from build123d import *

# Parameters (mm, degrees)
SKETCH1_W           = 54.7
SKETCH1_H           = 54.7
BOSS_EXTRUDE1_DEPTH = 6.35
SKETCH2_W           = 6.35
SKETCH2_H           = 13.5
SKETCH2_H_2         = 6.35
SKETCH2_W_2         = 13.5
CUT_EXTRUDE1_DEPTH  = 40.196524081


with BuildPart() as part:
    # Sketch1 → Boss-Extrude1 (new body)
    with BuildSketch(Plane.XY):
        Rectangle(SKETCH1_W, SKETCH1_H)
    extrude(amount=BOSS_EXTRUDE1_DEPTH)

    # Sketch2 → Cut-Extrude1 (cut, through all)
    with BuildSketch(Plane.XY.offset(6.35)):
        with Locations((-24.175, 14.25)):
            Rectangle(SKETCH2_W, SKETCH2_H)
        with Locations((-24.175, 24.175)):
            Rectangle(SKETCH2_W, SKETCH2_H_2)
        with Locations((-14.25, 24.175)):
            Rectangle(SKETCH2_W_2, SKETCH2_H_2)
        with Locations((14.25, 24.175)):
            Rectangle(SKETCH2_W_2, SKETCH2_H_2)
        with Locations((24.175, 24.175)):
            Rectangle(SKETCH2_W, SKETCH2_H_2)
        with Locations((24.175, 14.25)):
            Rectangle(SKETCH2_W, SKETCH2_H)
        with Locations((24.175, -14.25)):
            Rectangle(SKETCH2_W, SKETCH2_H)
        with Locations((24.175, -24.175)):
            Rectangle(SKETCH2_W, SKETCH2_H_2)
        with Locations((14.25, -24.175)):
            Rectangle(SKETCH2_W_2, SKETCH2_H_2)
        with Locations((-14.25, -24.175)):
            Rectangle(SKETCH2_W_2, SKETCH2_H_2)
        with Locations((-24.175, -24.175)):
            Rectangle(SKETCH2_W, SKETCH2_H_2)
        with Locations((-24.175, -14.25)):
            Rectangle(SKETCH2_W, SKETCH2_H)
    extrude(amount=-CUT_EXTRUDE1_DEPTH, mode=Mode.SUBTRACT)


solid = part.part
Here's how the part is built. I have some questions about the finished solid (model axes, mm). A direction names the side the tool comes from. Give positions to 0.01 mm unless a question says otherwise; leave off trailing zeros. Loops run counter-clockwise (first coordinate to the right, second up) from the corner with the lowest first, then second, coordinate; pieces in that order, holes last. Notation, with made-up numbers: (-21.75, -7) -> (2.25, -7) arc R22 cw to (2.25, 19) -> close; hole circle Ø3 at (55.25, 43.25). An arc over 180 degrees is marked (long way). Answer as a JSON object with one key per item and string values. Group by question number.
Item 1: I need wall thicknesses on L1, parallel to X at y = -11.5, z = 2; L2, parallel to X at y = 22, z = 4.5. Which ranges of each line are inside material? Lowest first, please.
Item 2: Imagine slicing it at B-B on y = 17. Write out the boundary of the cut face in (x, z).
Item 3: On a 3-axis mill with a long thin cutter (end or side, diameter ignored), from which of +Z, -Z, +X, -X, +Y, -Y can I reach the whole of each face in a straight line? I mean faces 1 (the flat face through (14, -21, 3)), 2 (the flat face through (-24, 7.5, 3)), 3 (the flat face through (-14, -21, 3)), 4 (the flat face through (24, 7.5, 3)), 5 (the flat face through (27.35, 0, 3)). Say none if no direction works.
Item 4: Will these pins go through, and if not, where does the flat tip stop? pin 1 (3 mm diameter, centred on y = -25, z = 3, fed in from -X); pin 2 (1.9 mm diameter, centred on y = 25.5, z = 4.5, fed in from +X); pin 3 (3 mm diameter, centred on y = -14, z = 4, fed in from -X).
Item 5: Imagine slicing it at A-A on z = 1.75. Write out the boundary of the cut face in (x, y).
Answer list:
{
 "1": {"L1": "x = -21 to 21", "L2": "x = -7.5 to 7.5"},
 "2": {"outline": "(-21, 0) -> (21, 0) -> (21, 6.35) -> (-21, 6.35) -> close"},
 "3": {"face 1": "+Z, -Z, +X, -Y", "face 2": "+Z, -Z, -X, +Y", "face 3": "+Z, -Z, -X, -Y", "face 4": "+Z, -Z, +X, +Y", "face 5": "+Z, -Z, +X, +Y, -Y"},
 "4": {"pin 1": "stops at x = -7.5", "pin 2": "stops at x = 7.5", "pin 3": "stops at x = -21"},
 "5": {"outline": "(-27.35, -7.5) -> (-21, -7.5) -> (-21, -21) -> (-7.5, -21) -> (-7.5, -27.35) -> (7.5, -27.35) -> (7.5, -21) -> (21, -21) -> (21, -7.5) -> (27.35, -7.5) -> (27.35, 7.5) -> (21, 7.5) -> (21, 21) -> (7.5, 21) -> (7.5, 27.35) -> (-7.5, 27.35) -> (-7.5, 21) -> (-21, 21) -> (-21, 7.5) -> (-27.35, 7.5) -> close"}
}
